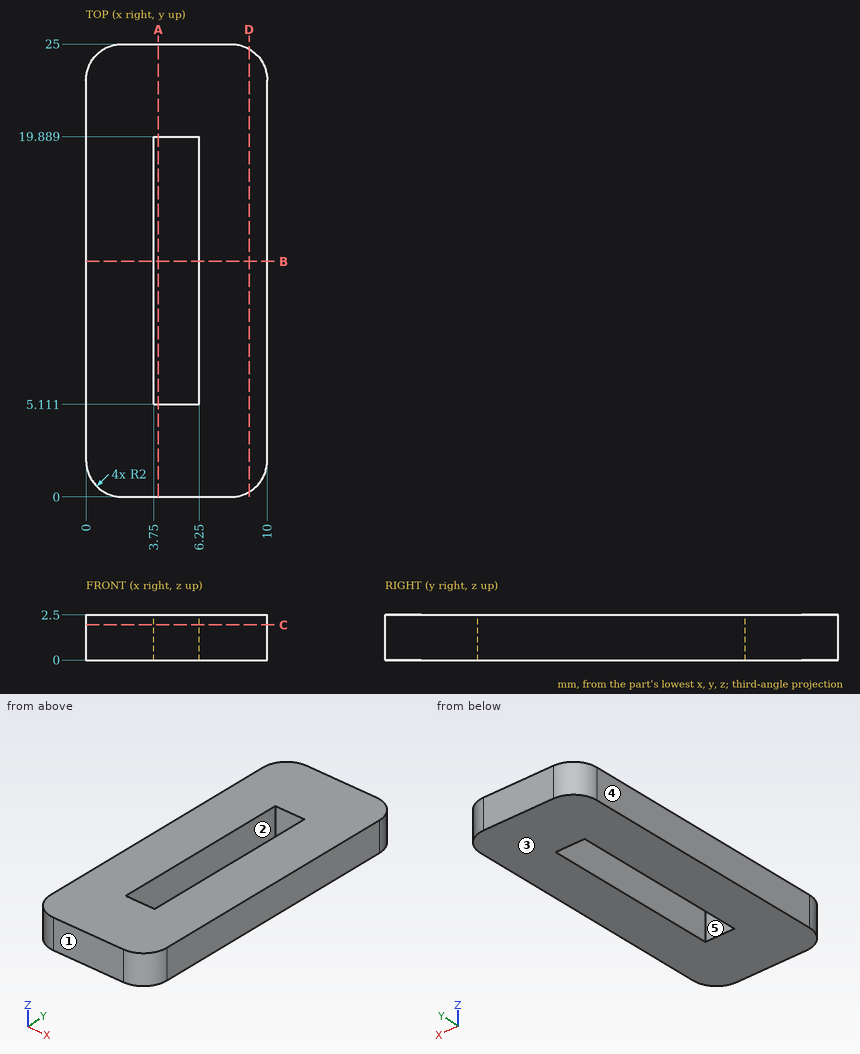
Answer from the drawing. Dimensions are ordinates in mm from the lowest x, y and z of the part. A direction names the side the tool comes from. Give positions to 0.01 mm unless a question says otherwise; leave off trailing zeros. Write each loop counter-clockwise with the first axis right and the second up, starting at its lowest first coordinate (ties: lowest second). Pieces come first, ordered by that corner, then holes.
1) A tool of negligible diameter and unlimited length cuts with its end or side. For the marked faces 1 and 2, from which of +Z, -Z, +X, -X, +Y, -Y can it reach the whole face along a straight path? Write none if from no direction.
2) Find the intervals of material crossed by L1, parallel to X at y = 18, z = 0.3; L2, parallel to Y at x = 5.25, z = 1.15; L3, parallel to Y at x = 9.75, z = 2.3 (1 decimal), in increasing order.
3) Section A-A (x = 4) is taken. Write down the section's boundary in (y, z).
4) Section C-C (z = 1.95) is taken. Write down the section's boundary in (x, y), and give its area (3 significant figures).
5) Section D-D (x = 9) is taken. Write down the section's boundary in (y, z).
6) For a pull along X with two mould halves and no side action, classify the marked faces 3, 4 and 5 as pulls with the +X half, pulls with the -X half, needs draft (parallel to the pull), parting line crosses it, or undercut.
7) Section B-B (y = 13) is taken. Write down the section's boundary in (x, z).
Response:
1. face 1: +Z, -Z, +X, -X, -Y
1. face 2: +Z, -Z
2. L1: x = 0 to 3.75, 6.25 to 10
2. L2: y = 0 to 5.11, 19.89 to 25
2. L3: y = 1 to 24
3. outline: (0, 0) - (5.11, 0) - (5.11, 2.5) - (0, 2.5) - close; (19.89, 0) - (25, 0) - (25, 2.5) - (19.89, 2.5) - close
4. outline: (0, 2) arc R2 ccw to (2, 0) - (8, 0) arc R2 ccw to (10, 2) - (10, 23) arc R2 ccw to (8, 25) - (2, 25) arc R2 ccw to (0, 23) - close; hole (3.75, 5.11) - (6.25, 5.11) - (6.25, 19.89) - (3.75, 19.89) - close
4. area: 210 mm2
5. outline: (0.27, 0) - (24.73, 0) - (24.73, 2.5) - (0.27, 2.5) - close
6. face 3: needs draft
6. face 4: pulls with the -X half
6. face 5: undercut
7. outline: (0, 0) - (3.75, 0) - (3.75, 2.5) - (0, 2.5) - close; (6.25, 0) - (10, 0) - (10, 2.5) - (6.25, 2.5) - close
